Geometry: see drawing. Coordinates: mm, zero at the bounding-box minimum. A direction names the side the tool comes from. Give positions to 0.01 mm unless a question says otherwise; leave off trailing zeros. Write each loop counter-clockwise with the first axis right and the second up, starting at its lowest first coordinate (ties: lowest second). Pieces come first, ordered by that corner, then holes.
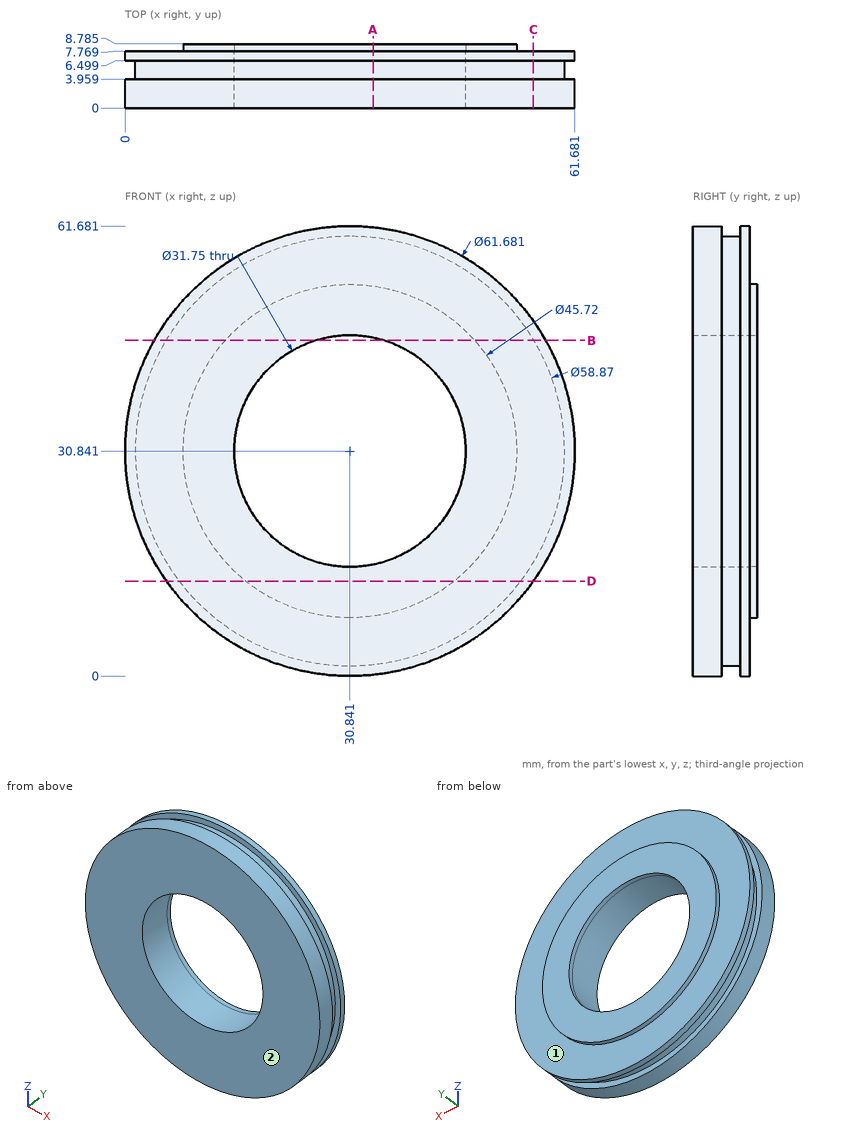
Q1. Section D-D, the plane z = 13. Return the cut outline in (x, y) (1 decimal), then the cut area to 3 significant figures.
Q2. Material intervals for line 1 along Y through (x, z) = (47.5, 55.5); line 2 along Y through (x, z) = (54, 22.5); line 3 along X through (y, z) = (7, 40) (1 decimal), sorted ascending.
Q3. Section C-C, the plane x = 56. Return the cut outline in (y, z).
Q4. Section B-B, the plane z = 46. Return the cut outline in (x, y) (1 decimal).
Q5. Access query for the marked faces 1 and 2. Directions: +Z, -Z, +X, -X, +Y, -Y. A direction counts if a zero-diameter tool reaches every point of the face in a straight line with its end or side. Return the directions, or none.
Q6. Pin query (flat end, axial travel): pin 1 (4 mm diameter, centred on y = 5, z = 34.5, fed in from -X); pin 2 (1 mm diameter, centred on x = 35.5, y = 2.5, fed in from +Z); pin 3 (3 mm diameter, centred on x = 53.5, z = 26, fed in from +Y) (1 decimal); pin 4 (2 mm diameter, centred on x = 17.5, y = 6, fed in from +Z). Return the tip coordinate at first contact, or that it passes through.
Q7. Section A-A, the plane x = 34. Return the cut outline in (y, z) (1 decimal).
Solutions:
1. outline: (5.7, 0) - (56, 0) - (56, 4) - (54.3, 4) - (54.3, 6.5) - (56, 6.5) - (56, 7.8) - (45.1, 7.8) - (45.1, 8.8) - (16.5, 8.8) - (16.5, 7.8) - (5.7, 7.8) - (5.7, 6.5) - (7.4, 6.5) - (7.4, 4) - (5.7, 4) - close
1. area: 411 mm2
2. line 1: y = 0 to 3.96, 6.5 to 7.77
2. line 2: y = 0 to 7.77
2. line 3: x = 1.4 to 17.9, 43.8 to 60.3
3. outline: (0, 13) - (3.96, 13) - (3.96, 15.56) - (6.5, 15.56) - (6.5, 13) - (7.77, 13) - (7.77, 48.68) - (6.5, 48.68) - (6.5, 46.12) - (3.96, 46.12) - (3.96, 48.68) - (0, 48.68) - close
4. outline: (4, 0) - (26.1, 0) - (26.1, 8.8) - (13.7, 8.8) - (13.7, 7.8) - (4, 7.8) - (4, 6.5) - (5.6, 6.5) - (5.6, 4) - (4, 4) - close; (35.6, 0) - (57.7, 0) - (57.7, 4) - (56.1, 4) - (56.1, 6.5) - (57.7, 6.5) - (57.7, 7.8) - (48, 7.8) - (48, 8.8) - (35.6, 8.8) - close
5. face 1: +Y
5. face 2: +Z, -Z, +X, -X, -Y
6. pin 1: stops at x = 0.06
6. pin 2: stops at z = 61.4
6. pin 3: stops at y = 8.8
6. pin 4: stops at z = 59.05
7. outline: (0, 0.2) - (4, 0.2) - (4, 1.6) - (6.5, 1.6) - (6.5, 0.2) - (7.8, 0.2) - (7.8, 8.2) - (8.8, 8.2) - (8.8, 15.3) - (0, 15.3) - close; (0, 46.4) - (8.8, 46.4) - (8.8, 53.5) - (7.8, 53.5) - (7.8, 61.5) - (6.5, 61.5) - (6.5, 60.1) - (4, 60.1) - (4, 61.5) - (0, 61.5) - close
